```python
from build123d import *

# Parameters (mm, degrees)
SKETCH1_R           = 37.5
SKETCH1_R_2         = 17.5
BOSS_EXTRUDE1_DEPTH = 76
SKETCH1_3_R         = 17.5
BOSS_EXTRUDE2_DEPTH = 78
SKETCH1_4_R         = 39
SKETCH1_4_R_2       = 37.5
BOSS_EXTRUDE3_DEPTH = 32
SKETCH2_R           = 1.75
CUT_EXTRUDE1_DEPTH  = 7
FILLET1_R           = 0.5
CHAMFER1_SIZE       = 0.5
CHAMFER2_SIZE       = 21.5
CHAMFER2_SIZE2      = 20
CHAMFER3_SIZE       = 1


with BuildPart() as part:
    # Sketch1 → Boss-Extrude1 (new body)
    with BuildSketch(Plane(origin=(0, 0, 0), x_dir=(1, 0, 0), z_dir=(0, 1, 0))):
        with Locations(Location((0, 0, 0), (0, 0, 270))):
            Circle(SKETCH1_R)
        with Locations(Location((0, 0, 0), (0, 0, 270))):
            Circle(SKETCH1_R_2, mode=Mode.SUBTRACT)
    extrude(amount=BOSS_EXTRUDE1_DEPTH)

    # Sketch1_3 → Boss-Extrude2 (add)
    with BuildSketch(Plane(origin=(0, 0, 0), x_dir=(1, 0, 0), z_dir=(0, 1, 0))):
        with Locations(Location((0, 0, 0), (0, 0, 270))):
            Circle(SKETCH1_3_R)
    extrude(amount=BOSS_EXTRUDE2_DEPTH)

    # Sketch1_4 → Boss-Extrude3 (add)
    with BuildSketch(Plane(origin=(0, 0, 0), x_dir=(1, 0, 0), z_dir=(0, 1, 0))):
        with Locations(Location((0, 0, 0), (0, 0, 270))):
            Circle(SKETCH1_4_R)
        with Locations(Location((0, 0, 0), (0, 0, 270))):
            Circle(SKETCH1_4_R_2, mode=Mode.SUBTRACT)
    extrude(amount=BOSS_EXTRUDE3_DEPTH)

    # Sketch2 → Cut-Extrude1 (cut)
    with BuildSketch(Plane(origin=(0, 76, 0), x_dir=(1, 0, 0), z_dir=(0, 1, 0))):
        with Locations(Location((0, 27.5, 0), (0, 0, 270))):
            Circle(SKETCH2_R)
        with Locations(Location((26.154054198, 8.497967345, 0), (0, 0, 270))):
            Circle(SKETCH2_R)
        with Locations(Location((16.164094438, -22.247967345, 0), (0, 0, 270))):
            Circle(SKETCH2_R)
        with Locations(Location((-16.164094438, -22.247967345, 0), (0, 0, 270))):
            Circle(SKETCH2_R)
        with Locations(Location((-26.154054198, 8.497967345, 0), (0, 0, 270))):
            Circle(SKETCH2_R)
    extrude(amount=-CUT_EXTRUDE1_DEPTH, mode=Mode.SUBTRACT)

    # Fillet1
    fillet1_edges = [part.edges().sort_by_distance(p)[0] for p in [
        (0, 32, -39),
    ]]
    fillet(fillet1_edges, radius=FILLET1_R)

    # Chamfer1
    chamfer1_edges = [part.edges().sort_by_distance(p)[0] for p in [
        (0, 76, -37.5),
    ]]
    chamfer(chamfer1_edges, length=CHAMFER1_SIZE)

    # Chamfer2
    chamfer2_edges = [part.edges().sort_by_distance(p)[0] for p in [
        (0, 0, -39),
    ]]
    chamfer2_side = [part.faces().sort_by_distance(p)[0] for p in [
        (0, 0, 0),
    ]]
    chamfer(chamfer2_edges, length=CHAMFER2_SIZE, length2=CHAMFER2_SIZE2, reference=chamfer2_side[0])

    # Chamfer3
    chamfer3_edges = [part.edges().sort_by_distance(p)[0] for p in [
        (0, 78, -17.5),
    ]]
    chamfer(chamfer3_edges, length=CHAMFER3_SIZE)


solid = part.part
```
Model file for the job. Use its own axes, mm. A direction names the side the tool comes from. Coordinates: 2 decimals unless noted, no trailing zeros. Write each loop counter-clockwise with the first axis right and the second up, starting at its lowest first coordinate (ties: lowest second). Pieces come first, ordered by that corner, then holes. Notation, with made-up numbers: (-27.75, 35.5) - (22.25, 35.5) arc R19 cw to (22.25, 47.5) - close; hole circle Ø1 at (81, 22.5). An arc over 180 degrees is marked (long way). One line per item, written item: value. Start each with the question number.
1. Slice it at C-C (y = 73.5). Write the cut outline in (x, z).
2. Flat gauge pins, fed straight in: pin 1 (4 mm diameter, centred on x = 0, z = -27.5, fed in from +Y); pin 2 (1 mm diameter, centred on y = 25, z = 8.5, fed in from -X); pin 3 (1.8 mm diameter, centred on x = 26.5, z = -9, fed in from +Y). Where does each tip first touch, or does it go through?
3. Tool access for faces 4 (the cylindrical face through (15.1, 72.55, 20.86)), 5 (the flat face through (0, 0, 0)): list every direction of +Z, -Z, +X, -X, +Y, -Y with a clear straight run to the whole face (end or side of a thin tool).
4. Slice it at B-B (z = 0). Write the cut outline in (x, y).
5. Slice it at D-D (y = 24.5). Write the cut outline in (x, z).
6. Mould opens along X. For faces 1 (the cylindrical face through (24.6, 72.55, -7.69)), 2 (the flat face through (-16, 76, 8)), 3 (the cylindrical face through (-10.648, 76.493, -13.887)) say: released by +X, released by -X, zero draft, split by the parting line, or undercut.
7. Probe line 1 (Z direction, x = 27.5, y = 73); line 2 (X direction, y = 26, z = -28); line 3 (X direction, y = 73, z = 11). List the from-to ranges inside material, lowest first. Write a range as from..to.
8. Slice it at A-A (x = 0). Write the cut outline in (y, z).
Answers below:
1. outline: circle Ø75 at (0, 0); hole circle Ø3.5 at (-26.15, -8.5); hole circle Ø3.5 at (-16.16, 22.25); hole circle Ø3.5 at (0, -27.5); hole circle Ø3.5 at (16.16, 22.25); hole circle Ø3.5 at (26.15, -8.5)
2. pin 1: stops at y = 76
2. pin 2: stops at x = -38.17
2. pin 3: stops at y = 69
3. face 4: +Y
3. face 5: +Z, -Z, +X, -X, -Y
4. outline: (-39, 20) - (-17.5, 0) - (17.5, 0) - (39, 20) - (39, 31.5) arc R0.5 ccw to (38.5, 32) - (37.5, 32) - (37.5, 75.5) - (37, 76) - (17.5, 76) - (17.5, 77) - (16.5, 78) - (-16.5, 78) - (-17.5, 77) - (-17.5, 76) - (-37, 76) - (-37.5, 75.5) - (-37.5, 32) - (-38.5, 32) arc R0.5 ccw to (-39, 31.5) - close
5. outline: circle Ø78 at (0, 0)
6. face 1: undercut
6. face 2: zero draft
6. face 3: split by the parting line
7. line 1: z = -25.5..-9.62, -7.38..25.5
7. line 2: x = -27.15..27.15
7. line 3: x = -35.85..35.85
8. outline: (0, -17.5) - (20, -39) - (31.5, -39) arc R0.5 ccw to (32, -38.5) - (32, -37.5) - (75.5, -37.5) - (76, -37) - (76, -29.25) - (69, -29.25) - (69, -25.75) - (76, -25.75) - (76, -17.5) - (77, -17.5) - (78, -16.5) - (78, 16.5) - (77, 17.5) - (76, 17.5) - (76, 37) - (75.5, 37.5) - (32, 37.5) - (32, 38.5) arc R0.5 ccw to (31.5, 39) - (20, 39) - (0, 17.5) - close
